```python
from build123d import *

# Parameters (mm, degrees)
F0_W     = 304.8
F0_H     = 152.4
F0_W_2   = 25.4
F0_H_2   = 101.6
F0_W_3   = 34.925
F1_DEPTH = 25.4
F2_DEPTH = 107.95
F4_DEPTH = 220.6635
F3_R     = 12.7
F5_DEPTH = 220.6635
F6_D     = 25.4


# Not quite as in the source:
# - a feature names something its author has since deleted; it is built from what else it names


with BuildPart() as f1:
    # F0 (on Top) → F1 (new body)
    with BuildSketch(Plane.XY):
        Rectangle(F0_W, F0_H)
        with Locations((-55.5625, 0)):
            Rectangle(F0_W_2, F0_H_2, mode=Mode.SUBTRACT)
        Rectangle(F0_W_3, F0_H_2, mode=Mode.SUBTRACT)
        with Locations((55.5625, 0)):
            Rectangle(F0_W_2, F0_H_2, mode=Mode.SUBTRACT)
        Rectangle(F0_W_3, F0_H_2)
        with Locations((-55.5625, 0)):
            Rectangle(F0_W_2, F0_H_2)
        with Locations((55.5625, 0)):
            Rectangle(F0_W_2, F0_H_2)
    extrude(amount=-F1_DEPTH)

    # F0 (on Top) → F2 (join)
    with BuildSketch(Plane.XY):
        with Locations((55.5625, 0)):
            Rectangle(F0_W_2, F0_H_2)
        Rectangle(F0_W_3, F0_H_2)
        with Locations((-55.5625, 0)):
            Rectangle(F0_W_2, F0_H_2)
    extrude(amount=F2_DEPTH)

    # F3 (on face) → F4 (cut, through all)
    with BuildSketch(Plane.YZ.offset(68.2625)):
        with BuildLine():
            Line((1e-10, 107.95), (-50.8, 107.95))
            Line((-50.8, 107.95), (-50.8, 57.15))
            ThreePointArc((-50.8, 57.15), (-35.9210244842, 93.0710244843), (1e-10, 107.95))
        make_face()
        with BuildLine():
            Line((50.8, 107.95), (1e-10, 107.95))
            ThreePointArc((1e-10, 107.95), (35.9210244843, 93.0710244842), (50.8, 57.15))
            Line((50.8, 57.15), (50.8, 107.95))
        make_face()
    extrude(amount=-F4_DEPTH, mode=Mode.SUBTRACT)

    # F3 (on face) → F5 (cut, through all)
    with BuildSketch(Plane.YZ.offset(68.2625)):
        with Locations((0, 76.2)):
            Circle(F3_R)
    extrude(amount=-F5_DEPTH, mode=Mode.SUBTRACT)

    # F6 (through all)
    with Locations(Plane.XY):
        with Locations((127, -50.8), (127, 50.8), (-127, 50.8), (-127, -50.8)):
            Hole(F6_D / 2)


solid = f1.part
```
Model file for the job. Use its own axes, mm. A direction names the side the tool comes from. Give positions to 0.01 mm unless a question says otherwise; leave off trailing zeros. Write each loop counter-clockwise with the first axis right and the second up, starting at its lowest first coordinate (ties: lowest second). Pieces come first, ordered by that corner, then holes. Notation, with made-up numbers: (40.5, -18.5) -> (89.5, -18.5) arc R6 ccw to (89.5, -13.5) -> close; hole circle Ø4 at (80.25, 60). An arc over 180 degrees is marked (long way). Use CSV: the item, a comma, the result in double quotes. Start each with the question number.
1) Tool access for faces 1 (the flat face through (-68.262, -1, 53)), 2 (the flat face through (68.262, -1, 53)), 3 (the flat face through (42.862, -1, 53)), 4 (the flat face through (-56, -50.8, 28)), 5 (the flat face through (0, 50.8, 28)): list every direction of +Z, -Z, +X, -X, +Y, -Y with a clear straight run to the whole face (end or side of a thin tool).
2) Cut at C-C on z = -8. List the corners of the cut face in (x, y), plus the area to 3 significant figures.
3) Cut at A-A on z = 29. List the corners of the cut face in (x, y), plus the area to 3 significant figures.
4) Cut at D-D on x = 14. List the corners of the cut face in (y, z), plus the area to 3 significant figures.
5) Two-plate mould, pull along X, no slides. Class faces 6 (the flat face through (152.4, -1, -13)), 7 (the flat face through (17.462, -1, 53)), 8 (the flat face through (55, 50.8, 28)): released by +X, released by -X, zero draft, split by the parting line, or undercut.
6) Drill centre lines: L1, parallel to X at y = 0, z = 96.5; L2, parallel to X at y = -50, z = -9; L3, parallel to Z at x = -34.5, y = -67.5. Where is each one in solid material? Low to high.
7) Cut at B-B on x = -127. List the corners of the cut face in (y, z), plus the area to 3 significant figures.
8) Pin check, flat tips, straight feed: P1, Ø2, axis at y = -51, z = 43.5, coming from the -X side; P2, Ø1, axis at x = -70, z = 10.5, coming from the -Y side; P3, Ø10, axis at y = -45.5, z = 64.5, coming from the +X side; P4, Ø12.5, axis at x = 55.5, z = 23, coming from the +Y side. Stop position of each tip, or through.
Final values:
1,face 1,"+Z, -X, +Y, -Y"
1,face 2,"+Z, +X, +Y, -Y"
1,face 3,"+Z, +Y, -Y"
1,face 4,"+Z, +X, -X, -Y"
1,face 5,"+Z, +X, -X, +Y"
2,outline,"(-152.4, -76.2) -> (152.4, -76.2) -> (152.4, 76.2) -> (-152.4, 76.2) -> close; hole circle Ø25.4 at (-127, -50.8); hole circle Ø25.4 at (-127, 50.8); hole circle Ø25.4 at (127, -50.8); hole circle Ø25.4 at (127, 50.8)"
2,area,"44,400 mm2"
3,outline,"(-68.26, -50.8) -> (-42.86, -50.8) -> (-42.86, 50.8) -> (-68.26, 50.8) -> close; (-17.46, -50.8) -> (17.46, -50.8) -> (17.46, 50.8) -> (-17.46, 50.8) -> close; (42.86, -50.8) -> (68.26, -50.8) -> (68.26, 50.8) -> (42.86, 50.8) -> close"
3,area,"8,710 mm2"
4,outline,"(-76.2, -25.4) -> (76.2, -25.4) -> (76.2, 0) -> (50.8, 0) -> (50.8, 57.15) arc R50.8 ccw to (-50.8, 57.15) -> (-50.8, 0) -> (-76.2, 0) -> close; hole circle Ø25.4 at (0, 76.2)"
4,area,"13,200 mm2"
5,face 6,"released by +X"
5,face 7,"undercut"
5,face 8,"zero draft"
6,L1,"x = -68.26 to -42.86, -17.46 to 17.46, 42.86 to 68.26"
6,L2,"x = -152.4 to -139.67, -114.33 to 114.33, 139.67 to 152.4"
6,L3,"z = -25.4 to 0"
7,outline,"(-76.2, -25.4) -> (-63.5, -25.4) -> (-63.5, 0) -> (-76.2, 0) -> close; (-38.1, -25.4) -> (38.1, -25.4) -> (38.1, 0) -> (-38.1, 0) -> close; (63.5, -25.4) -> (76.2, -25.4) -> (76.2, 0) -> (63.5, 0) -> close"
7,area,"2,580 mm2"
8,P1,"stops at x = -68.26"
8,P2,"passes through"
8,P3,"stops at x = 68.26"
8,P4,"stops at y = 50.8"
